Here's how the part is built. I have some questions about the finished solid (model axes, mm). Face numbers are marked on the shaded views. Round coordinates to 2 decimals unless told otherwise and drop trailing zeros. Write each loop counter-clockwise with the first axis right and the second up, starting at its lowest first coordinate (ties: lowest second). Pieces come first, ordered by that corner, then holes. Notation, with made-up numbers: (25.5, 45) -> (69.5, 45) arc R20 cw to (69.5, 68) -> close; hole circle Ø1 at (54.5, -22). An arc over 180 degrees is marked (long way). Answer in a Markdown table with one row per item.
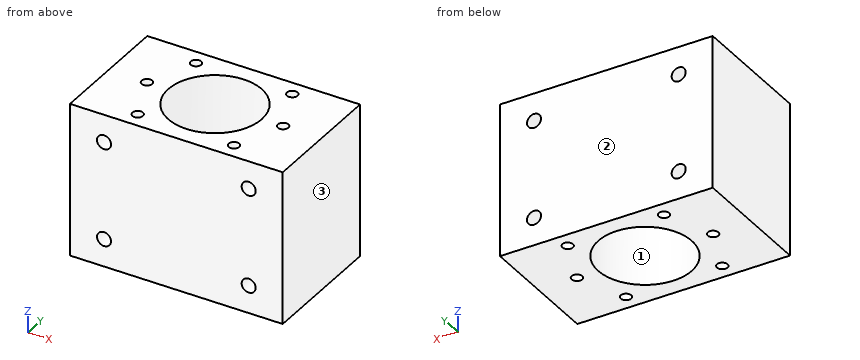
from build123d import *

# Parameters (mm, degrees)
SKETCH_1_W         = 50
SKETCH_1_H         = 30
SKETCH_1_R         = 11
EXTRUDE_1_DEPTH    = 18
HOLE_WIZARD_M3_1_D = 2.5
HOLE_WIZARD_M4_1_D = 3.3
MIRROR_2_COPY_1_D  = 3.3


with BuildPart() as part:
    # 草图1 → 凸台-拉伸1 (new, symmetric)
    with BuildSketch(Plane.XY):
        Rectangle(SKETCH_1_W, SKETCH_1_H)
        Circle(SKETCH_1_R, mode=Mode.SUBTRACT)
    extrude(amount=EXTRUDE_1_DEPTH, both=True)

    # M3 螺纹孔的螺纹孔钻头1 (through all)
    with Locations(Plane(origin=(-16, 0, 18), x_dir=(1, 0, 0), z_dir=(0, 0, 1))):
        with Locations((0, 0), (4.686291501, 11.313708499), (27.313708499, 11.313708499), (32, 0), (27.313708499, -11.313708499), (4.686291501, -11.313708499)):
            Hole(HOLE_WIZARD_M3_1_D / 2)

    # M4 螺纹孔的螺纹孔钻头1 (through all)
    with Locations(Plane(origin=(-17, 15, -11.5), x_dir=(0, 0, 1), z_dir=(0, 1, 0))):
        with Locations((0, 0)):
            hole_wizard_m4_1 = Hole(HOLE_WIZARD_M4_1_D / 2)

    # 镜向1: M4 螺纹孔的螺纹孔钻头1 across plane
    add(hole_wizard_m4_1.mirror(Plane(origin=(0, 0, 0), x_dir=(0, 0, 1), z_dir=(1, 0, 0))), mode=Mode.SUBTRACT)

    # 镜向2: M4 螺纹孔的螺纹孔钻头1 across plane
    add(hole_wizard_m4_1.mirror(Plane.XY), mode=Mode.SUBTRACT)

    # 镜向2 copy 1 (through all)
    with Locations(Plane(origin=(17, 15, 11.5), x_dir=(0, 0, -1), z_dir=(0, 1, 0))):
        with Locations((0, 0)):
            Hole(MIRROR_2_COPY_1_D / 2)


solid = part.part
1) I want a section at A-A, the plane x = 0. List the corners of the cut face in (y, z) for me, and give its area (3 significant figures).
Response:
| item | result |
|---|---|
| outline | (-15, -18) -> (-11, -18) -> (-11, 18) -> (-15, 18) -> close; (11, -18) -> (15, -18) -> (15, 18) -> (11, 18) -> close |
| area | 288 mm^2 |
2) I want a section at D-D, the plane x = 16. List the corners of the cut face in (y, z) for me.
Response:
| item | result |
|---|---|
| outline | (-15, -18) -> (-1.25, -18) -> (-1.25, -12.81) -> (-15, -12.81) -> close; (-15, -10.19) -> (-1.25, -10.19) -> (-1.25, 10.19) -> (-15, 10.19) -> close; (-15, 12.81) -> (-1.25, 12.81) -> (-1.25, 18) -> (-15, 18) -> close; (1.25, -18) -> (15, -18) -> (15, -12.81) -> (1.25, -12.81) -> close; (1.25, -10.19) -> (15, -10.19) -> (15, 10.19) -> (1.25, 10.19) -> close; (1.25, 12.81) -> (15, 12.81) -> (15, 18) -> (1.25, 18) -> close |
3) I want a section at C-C, the plane z = -11.5. List the corners of the cut face in (x, y) for me.
Response:
| item | result |
|---|---|
| outline | (-25, -15) -> (-18.65, -15) -> (-18.65, 15) -> (-25, 15) -> close; (-15.35, -15) -> (15.35, -15) -> (15.35, -1.07) arc R1.25 cw to (15.35, 1.07) -> (15.35, 15) -> (-15.35, 15) -> (-15.35, 1.07) arc R1.25 cw to (-15.35, -1.07) -> close; (18.65, -15) -> (25, -15) -> (25, 15) -> (18.65, 15) -> close; hole circle Ø2.5 at (-11.31, -11.31); hole circle Ø2.5 at (-11.31, 11.31); hole circle Ø22 at (0, 0); hole circle Ø2.5 at (11.31, -11.31); hole circle Ø2.5 at (11.31, 11.31) |
4) We'd pull the mould along Y, two halves only. Please class the marked faces 1, 2 and 3: +Y half, -Y half, draft (parallel to the pull), parting line (faces both ways), or undercut.
Response:
| item | result |
|---|---|
| face 1 | undercut |
| face 2 | +Y half |
| face 3 | draft |
5) I want a section at B-B, the plane y = 3. List the corners of the cut face in (x, z) for me.
Response:
| item | result |
|---|---|
| outline | (-25, -18) -> (-10.58, -18) -> (-10.58, 18) -> (-25, 18) -> close; (10.58, -18) -> (25, -18) -> (25, 18) -> (10.58, 18) -> close; hole circle Ø3.3 at (-17, -11.5); hole circle Ø3.3 at (-17, 11.5); hole circle Ø3.3 at (17, -11.5); hole circle Ø3.3 at (17, 11.5) |
6) I need wall thicknesses on line 1 (X direction, y = 11.5, z = 15); line 2 (Z direction, x = 17, y = -2); line 3 (X direction, y = -5, z = 11). Which ranges of each line are inside material? Lowest first, please. Write a range as [from, to].
Response:
| item | result |
|---|---|
| line 1 | x = [-25, -12.55], [-10.08, 10.08], [12.55, 25] |
| line 2 | z = [-18, -13.15], [-9.85, 9.85], [13.15, 18] |
| line 3 | x = [-25, -18.57], [-15.43, -9.8], [9.8, 15.43], [18.57, 25] |
